```python
from build123d import *

# Parameters (mm, degrees)
SKETCH1_W                                         = 152.4
SKETCH1_H                                         = 25.4
SKETCH1_R                                         = 4.7625
BOSS_EXTRUDE1_DEPTH                               = 6.35
CSK_FOR_6_FLAT_HEAD_MACHINE_SCREW_100_D           = 3.7973
CSK_FOR_6_FLAT_HEAD_MACHINE_SCREW_100_CSINK_D     = 7.0866
CSK_FOR_6_FLAT_HEAD_MACHINE_SCREW_100_CSINK_ANGLE = 100
SKETCH5_W                                         = 6.35
SKETCH5_H                                         = 1.5875
CUT_EXTRUDE1_DEPTH                                = 116.178567885
MIRROR2_COPY_1_SKETCH_W                           = 6.35
MIRROR2_COPY_1_SKETCH_H                           = 1.5875
MIRROR2_COPY_1_DEPTH                              = 116.178567885


with BuildPart() as part:
    # Sketch1 → Boss-Extrude1 (new body)
    with BuildSketch(Plane.XY):
        with Locations((-38.1, 0)):
            Rectangle(SKETCH1_W, SKETCH1_H)
        Polygon((-95.538789083, -9.525), (-57.15, -1.298830911), (-18.761210917, -9.525), align=None, mode=Mode.SUBTRACT)
        Polygon((23.87364996, -9.525), (14.22635004, -9.525), (19.05, -2.28952506), align=None, mode=Mode.SUBTRACT)
        Polygon((-101.6, 8.226169089), (-63.211210917, 0), (-101.6, -8.226169089), align=None, mode=Mode.SUBTRACT)
        Polygon((-18.761210917, 9.525), (-57.15, 1.298830911), (-95.538789083, 9.525), align=None, mode=Mode.SUBTRACT)
        Polygon((-12.7, -8.226169089), (-51.088789083, 0), (-12.7, 8.226169089), align=None, mode=Mode.SUBTRACT)
        Circle(SKETCH1_R, mode=Mode.SUBTRACT)
        Polygon((17.52364996, 0), (12.7, -7.23547494), (12.7, 7.23547494), align=None, mode=Mode.SUBTRACT)
        Polygon((25.4, 7.23547494), (25.4, -7.23547494), (20.57635004, 0), align=None, mode=Mode.SUBTRACT)
        Polygon((19.05, 2.28952506), (14.22635004, 9.525), (23.87364996, 9.525), align=None, mode=Mode.SUBTRACT)
    extrude(amount=BOSS_EXTRUDE1_DEPTH)

    # CSK for _6 Flat Head Machine Screw _100 (through all)
    with Locations(Plane(origin=(0, 0, 0), x_dir=(-1, 0, 0), z_dir=(0, 0, -1))):
        with Locations((-34.925, 6.35), (-34.925, -6.35), (111.125, -6.35), (111.125, 6.35)):
            CounterSinkHole(CSK_FOR_6_FLAT_HEAD_MACHINE_SCREW_100_D / 2, CSK_FOR_6_FLAT_HEAD_MACHINE_SCREW_100_CSINK_D / 2, counter_sink_angle=CSK_FOR_6_FLAT_HEAD_MACHINE_SCREW_100_CSINK_ANGLE)

    # Sketch5 → Cut-Extrude1 (cut, through all)
    with BuildSketch(Plane(origin=(0, 0, 0), x_dir=(-1, 0, 0), z_dir=(0, 0, -1))):
        with Locations((111.125, -11.90625)):
            Rectangle(SKETCH5_W, SKETCH5_H)
    cut_extrude1 = extrude(amount=-CUT_EXTRUDE1_DEPTH, mode=Mode.SUBTRACT)

    # Mirror1: Cut-Extrude1 across plane
    add(cut_extrude1.mirror(Plane.ZY.offset(38.1)), mode=Mode.SUBTRACT)

    # Mirror2: Cut-Extrude1 across plane
    add(cut_extrude1.mirror(Plane(origin=(0, 0, 0), x_dir=(0, 0, 1), z_dir=(0, -1, 0))), mode=Mode.SUBTRACT)

    # Mirror2 copy 1 sketch → Mirror2 copy 1 (cut, through all)
    with BuildSketch(Plane(origin=(-76.2, 0, 0), x_dir=(1, 0, 0), z_dir=(0, 0, -1))):
        with Locations((111.125, -11.90625)):
            Rectangle(MIRROR2_COPY_1_SKETCH_W, MIRROR2_COPY_1_SKETCH_H)
    extrude(amount=-MIRROR2_COPY_1_DEPTH, mode=Mode.SUBTRACT)


solid = part.part
```
Read the model definition and answer for the solid it produces. Units are mm, in the model's axes. A direction names the side the tool comes from. Round coordinates to 2 decimals unless told otherwise and drop trailing zeros. Write each loop counter-clockwise with the first axis right and the second up, starting at its lowest first coordinate (ties: lowest second). Pieces come first, ordered by that corner, then holes. Notation, with made-up numbers: (82, 20.25) -> (99, 20.25) arc R25 ccw to (99, 52.25) -> close; hole circle Ø9 at (-9, -33). An arc over 180 degrees is marked (long way). Answer in a Markdown table with one row per item. Add a question column.
1) Find section A-A, the plane x = 0. Determine the outline of the cut face in (y, z).
2) Given P1, Ø0.8, axis at y = -12.5, z = 1.5, coming from the -X side; P2, Ø0.5, axis at y = -12, z = 4, coming from the +X side; P3, Ø3, axis at x = 33.5, z = 2.5, coming from the -Y side, each flat-ended and moving along its own axis, determine where each tip first touches the part or whether it passes through.
3) Which of the six approach directions +Z, -Z, +X, -X, +Y, -Y give full straight-line access (tool end or side, diameter ignored) to faces 1 (the face through (-111, 11.112, 3)), 2 (the face through (21.496, 5.958, 3.131)), 3 (the face through (33, -5, 1))?
4) Find section C-C, the plane x = -85.5. Determine the outline of the cut face in (y, z) (3 decimals).
5) Find section B-B, the plane z = 3.5. State how many separate pieces and enclosed holes the cut face has, and give its area (3 significant figures).
6) Consider line 1 (Y direction, x = -97, z = 2.5); line 2 (Y direction, x = 0, z = 3.25); line 3 (Y direction, x = -46.5, z = 2.5) (3 decimals). Determine where each line is inside the solid, lowest interval first.
7) Determine the mould class of faces 4 (the face through (-39, -12.7, 3)), 5 (the face through (38.1, 0, 3)), 6 (the face through (-82.137, -4.056, 3.131)) for opening direction Y: pulls with the +Y half, pulls with the -Y half, needs draft (parallel to the pull), parting line crosses it, or undercut.
Findings below:
| question | item | result |
|---|---|---|
| 1 | outline | (-12.7, 0) -> (-4.76, 0) -> (-4.76, 6.35) -> (-12.7, 6.35) -> close; (4.76, 0) -> (12.7, 0) -> (12.7, 6.35) -> (4.76, 6.35) -> close |
| 2 | P1 | x = -107.95 |
| 2 | P2 | x = 31.75 |
| 2 | P3 | y = -11.11 |
| 3 | face 1 | +Z, -Z, -X, +Y |
| 3 | face 2 | +Z, -Z |
| 3 | face 3 | -Z |
| 4 | outline | (-12.7, 0) -> (-9.525, 0) -> (-9.525, 6.35) -> (-12.7, 6.35) -> close; (-7.374, 0) -> (-4.776, 0) -> (-4.776, 6.35) -> (-7.374, 6.35) -> close; (4.776, 0) -> (7.374, 0) -> (7.374, 6.35) -> (4.776, 6.35) -> close; (9.525, 0) -> (12.7, 0) -> (12.7, 6.35) -> (9.525, 6.35) -> close |
| 5 | separate pieces | 1 |
| 5 | enclosed holes | 13 |
| 5 | area | 2,310 mm² |
| 6 | line 1 | -12.7 to -7.24, 7.24 to 12.7 |
| 6 | line 2 | -12.7 to -4.76, 4.76 to 12.7 |
| 6 | line 3 | -12.7 to -9.525, -3.581 to -0.983, 0.983 to 3.581, 9.525 to 12.7 |
| 7 | face 4 | pulls with the -Y half |
| 7 | face 5 | needs draft |
| 7 | face 6 | undercut |
